Build history of the part. All positions in model axes, mm. Give positions to 0.01 mm unless a question says otherwise; leave off trailing zeros. Order: outer loops, then holes, each group sorted by start corner. A loop starts at its lowest first (then second) coordinate and runs counter-clockwise, first axis right, second up. Notation, with made-up numbers: (69.25, 46.5) -> (78.25, 46.5) arc R14 cw to (78.25, 58.5) -> close; hole circle Ø3 at (57, -37.75). An arc over 180 degrees is marked (long way). Use a Markdown table: item, result. Add a question column.
Autodesk Inventor part; units mm, degrees
ref_plane "YZ Plane" through (0, 0, 0) normal (1, 0, 0) x (0, 1, 0)
ref_plane "XZ Plane" through (0, 0, 0) normal (0, 1, 0) x (-1, 0, 0)
ref_plane "XY Plane" through (0, 0, 0) normal (0, 0, 1) x (1, 0, 0)
sketch "Sketch1" plane through (0, 0, 0) normal (0, 0, 1) x (1, 0, 0)
  line L0 (0, 0) -> (7, 0)
  line L1 (7, 0) -> (7, 20)
  line L2 (7, 20) -> (0, 20)
  line L3 (0, 20) -> (0, 0)
  dimension "d0" = 7
  dimension "d1" = 20
extrude "Extrusion1" add sketch "Sketch1" along normal blind 3
fillet "Fillet1" radius 3.5 4 edges at (0, 0, 1.5) (7, 0, 1.5) (0, 20, 1.5) (7, 20, 1.5)
sketch "Sketch2" plane through (0, 0, 3) normal (0, 0, 1) x (1, 0, 0)
  arc A0 (7, 16.5) -> (0, 16.5) centre (3.5, 16.5) ccw
  arc A1 (0, 3.5) -> (7, 3.5) centre (3.5, 3.5) ccw
hole "Hole1" at (3.5, 3.5, 3) at (3.5, 16.5, 3) direction (0, 0, -1) diameter 3 end through all
properties part number "plastic_part_13"
(1) Band-saw the part on C-C on x = 3.25. Give the cut face in (y, z), plus the area to 3 significant figures.
(2) Band-saw the part on B-B on x = 4.25. Give the cut face in (y, z), plus the area to 3 significant figures.
(3) Band-saw the part on A-A on z = 1.6. State how many separate pieces and enclosed holes the cut face has, plus the area to 3 significant figures.
(4) Pin check, flat tips, straight feed: pin 1 Ø1.5 at (x, z) = (0.5, 2) entering from -Y; pin 2 Ø2.5 at (x, y) = (3.5, 3.5) entering from +Z. Stop position of each tip, or through.
(5) Wall check: probe 1 along Y at (x, z) = (3.5, 0.65); probe 2 along Y at (x, z) = (4, 0.45); probe 3 along X at (y, z) = (3.5, 1.25). Give the ranges that are in metal, low to high.
(6) Band-saw the part on D-D on y = 18.5. Give the cut face in (x, z), plus the area to 3 significant figures.
Response:
| question | item | result |
|---|---|---|
| 1 | outline | (0.01, 0) -> (2.02, 0) -> (2.02, 3) -> (0.01, 3) -> close; (4.98, 0) -> (15.02, 0) -> (15.02, 3) -> (4.98, 3) -> close; (17.98, 0) -> (19.99, 0) -> (19.99, 3) -> (17.98, 3) -> close |
| 1 | area | 42.2 mm² |
| 2 | outline | (0.08, 0) -> (2.2, 0) -> (2.2, 3) -> (0.08, 3) -> close; (4.8, 0) -> (15.2, 0) -> (15.2, 3) -> (4.8, 3) -> close; (17.8, 0) -> (19.92, 0) -> (19.92, 3) -> (17.8, 3) -> close |
| 2 | area | 43.9 mm² |
| 3 | separate pieces | 1 |
| 3 | enclosed holes | 2 |
| 3 | area | 115 mm² |
| 4 | pin 1 | stops at y = 0.82 |
| 4 | pin 2 | passes through |
| 5 | probe 1 | y = 0 to 2, 5 to 15, 18 to 20 |
| 5 | probe 2 | y = 0.04 to 2.09, 4.91 to 15.09, 17.91 to 19.96 |
| 5 | probe 3 | x = 0 to 2, 5 to 7 |
| 6 | outline | (0.63, 0) -> (6.37, 0) -> (6.37, 3) -> (0.63, 3) -> close |
| 6 | area | 17.2 mm² |
